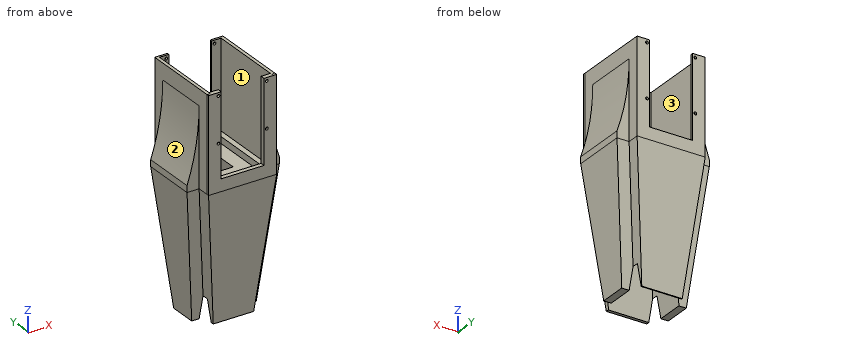
```python
from build123d import *
from build123d.topology import SkipClean

# Parameters (mm, degrees)
BOSS_EXTRUDE1_DEPTH      = 3
SKETCH2_W                = 25
SKETCH2_H                = 2
BOSS_EXTRUDE2_DEPTH      = 40
SKETCH3_R                = 0.625
CUT_EXTRUDE1_DEPTH       = 3
SKETCH4_R                = 0.625
CUT_EXTRUDE2_DEPTH       = 3
SKETCH7_W                = 19.5
SKETCH7_H                = 75
CUT_EXTRUDE5_DEPTH       = 40
SKETCH10_W               = 25
SKETCH10_H               = 3
BOSS_EXTRUDE4_DEPTH      = 10
SKETCH11_W               = 25
SKETCH11_H               = 3
BOSS_EXTRUDE5_DEPTH      = 10
SKETCH12_W               = 3
SKETCH12_H               = 25
BOSS_EXTRUDE6_DEPTH      = 10
SKETCH13_W               = 3
SKETCH13_H               = 25
BOSS_EXTRUDE7_DEPTH      = 10
SKETCH14_W               = 43
SKETCH14_H               = 35.95813892
BOSS_EXTRUDE11_DEPTH     = 3
SKETCH15_W               = 43
SKETCH15_H               = 35.95813892
BOSS_EXTRUDE12_DEPTH     = 3
SKETCH16_W               = 23
SKETCH16_H               = 28
CUT_EXTRUDE6_DEPTH       = 13
FILLET1_R                = 10
FILLET2_R                = 10
SKETCH19_W               = 28
SKETCH19_H               = 32
CUT_EXTRUDE9_DEPTH       = 40
CUT_EXTRUDE11_DEPTH      = 58.835974964
CUT_EXTRUDE11_DEPTH_BACK = 58.835974964
SKETCH20_W               = 25.25
SKETCH20_H               = 11.847644437
SKETCH20_W_2             = 25
SKETCH20_H_2             = 13.837487399
CUT_EXTRUDE13_DEPTH      = 56.982140009
CUT_EXTRUDE13_DEPTH_BACK = 56.982140009
SKETCH22_W               = 10
SKETCH22_H               = 25
FILLET3_R                = 100
FILLET4_R                = 100
SKETCH25_W               = 28
SKETCH25_H               = 2
CUT_EXTRUDE17_DEPTH      = 40
SKETCH27_R               = 0.625
BOSS_EXTRUDE14_DEPTH     = 1
SKETCH31_W               = 10
SKETCH31_H               = 10
BOSS_EXTRUDE16_DEPTH     = 60
BOSS_EXTRUDE16_TAPER     = 6


# Some blends are built 0.0001 mm under size
with BuildPart() as part:
    # Sketch1 → Boss-Extrude1 (new body)
    with BuildSketch(Plane.XY):
        Polygon((12.5, 12.5), (21, 12.5), (21, -12.5), (12.5, -12.5), (12.5, -18), (-12.5, -18), (-12.5, -12.5), (-21, -12.5), (-21, 12.5), (-12.5, 12.5), (-12.5, 18), (12.5, 18), align=None)
    extrude(amount=BOSS_EXTRUDE1_DEPTH)

    # Sketch2 → Boss-Extrude2 (add)
    with BuildSketch(Plane.XY.offset(3)):
        with Locations((0, 17)):
            Rectangle(SKETCH2_W, SKETCH2_H)
        with Locations((0, -17)):
            Rectangle(SKETCH2_W, SKETCH2_H)
    extrude(amount=BOSS_EXTRUDE2_DEPTH)

    # Sketch3 → Cut-Extrude1 (cut)
    with BuildSketch(Plane(origin=(0, 18, 0), x_dir=(1, 0, 0), z_dir=(0, 1, 0))):
        with Locations(Location((-11, -17.5, 0), (0, 0, 270))):
            Circle(SKETCH3_R)
        with Locations(Location((11, -17.5, 0), (0, 0, 270))):
            Circle(SKETCH3_R)
        with Locations(Location((-11, -41.5, 0), (0, 0, 270))):
            Circle(SKETCH3_R)
        with Locations(Location((11, -41.5, 0), (0, 0, 270))):
            Circle(SKETCH3_R)
    extrude(amount=-CUT_EXTRUDE1_DEPTH, mode=Mode.SUBTRACT)

    # Sketch4 → Cut-Extrude2 (cut)
    with BuildSketch(Plane(origin=(0, -16, 0), x_dir=(1, 0, 0), z_dir=(0, 1, 0))):
        with Locations(Location((-11, -41.5, 0), (0, 0, 270))):
            Circle(SKETCH4_R)
        with Locations(Location((11, -41.5, 0), (0, 0, 270))):
            Circle(SKETCH4_R)
        with Locations(Location((-11, -21, 0), (0, 0, 270))):
            Circle(SKETCH4_R)
        with Locations(Location((11, -21, 0), (0, 0, 270))):
            Circle(SKETCH4_R)
    extrude(amount=-CUT_EXTRUDE2_DEPTH, mode=Mode.SUBTRACT)

    # Sketch7 → Cut-Extrude5 (cut)
    with BuildSketch(Plane(origin=(0, 18, 0), x_dir=(1, 0, 0), z_dir=(0, 1, 0))):
        with Locations((0, -43)):
            Rectangle(SKETCH7_W, SKETCH7_H)
    extrude(amount=-CUT_EXTRUDE5_DEPTH, mode=Mode.SUBTRACT)

    # Sketch10 → Boss-Extrude4 (add)
    with BuildSketch(Plane(origin=(0, 18, 0), x_dir=(1, 0, 0), z_dir=(0, 1, 0))):
        with Locations((0, -1.5)):
            Rectangle(SKETCH10_W, SKETCH10_H)
    extrude(amount=BOSS_EXTRUDE4_DEPTH)

    # Sketch11 → Boss-Extrude5 (add)
    with BuildSketch(Plane.XZ.offset(18)):
        with Locations((0, 1.5)):
            Rectangle(SKETCH11_W, SKETCH11_H)
    extrude(amount=BOSS_EXTRUDE5_DEPTH)

    # Sketch12 → Boss-Extrude6 (add)
    with BuildSketch(Plane.ZY.offset(21)):
        with Locations((1.5, 0)):
            Rectangle(SKETCH12_W, SKETCH12_H)
    extrude(amount=BOSS_EXTRUDE6_DEPTH)

    # Sketch13 → Boss-Extrude7 (add)
    with BuildSketch(Plane(origin=(21, 0, 0), x_dir=(0, 0, -1), z_dir=(1, 0, 0))):
        with Locations((-1.5, 0)):
            Rectangle(SKETCH13_W, SKETCH13_H)
    extrude(amount=BOSS_EXTRUDE7_DEPTH)

    # Sketch14 → Boss-Extrude11 (add)
    with BuildSketch(Plane.ZY.offset(12.5)):
        with Locations((21.5, 0.02093054)):
            Rectangle(SKETCH14_W, SKETCH14_H)
    extrude(amount=BOSS_EXTRUDE11_DEPTH)

    # Sketch15 → Boss-Extrude12 (add)
    with BuildSketch(Plane(origin=(12.5, 0, 0), x_dir=(0, 0, -1), z_dir=(1, 0, 0))):
        with Locations((-21.5, 0.02093054)):
            Rectangle(SKETCH15_W, SKETCH15_H)
    extrude(amount=BOSS_EXTRUDE12_DEPTH)

    # Sketch16 → Cut-Extrude6 (cut)
    with BuildSketch(Plane(origin=(0, 0, 0), x_dir=(-1, 0, 0), z_dir=(0, 0, -1))):
        Rectangle(SKETCH16_W, SKETCH16_H)
    extrude(amount=-CUT_EXTRUDE6_DEPTH, mode=Mode.SUBTRACT)

    # Fillet1
    fillet1_edges = [part.edges().sort_by_distance(p)[0] for p in [
        (31, 12.5, 1.5),
    ]]
    fillet(fillet1_edges, radius=FILLET1_R)

    # Fillet2
    fillet2_edges = [part.edges().sort_by_distance(p)[0] for p in [
        (12.5, 28, 1.5),
        (-12.5, 28, 1.5),
        (-31, 12.5, 1.5),
        (12.5, -28, 1.5),
        (-31, -12.5, 1.5),
        (-12.5, -28, 1.5),
        (31, -12.5, 1.5),
    ]]
    fillet(fillet2_edges, radius=FILLET2_R - 0.0001)  # a hair under: the kernel refuses the full size

    # Sketch19 → Cut-Extrude9 (cut)
    with BuildSketch(Plane.XY.offset(43)):
        Rectangle(SKETCH19_W, SKETCH19_H)
    extrude(amount=-CUT_EXTRUDE9_DEPTH, mode=Mode.SUBTRACT)

    # Sketch20 → Cut-Extrude11 (cut, two sides: drawn at the far end of the back side and taken through both)
    with BuildSketch(Plane.XY.offset(3).offset(-CUT_EXTRUDE11_DEPTH_BACK)):
        with Locations((0, 23.923822218)):
            Rectangle(SKETCH20_W, SKETCH20_H)
        with Locations((0, -24.918743699)):
            Rectangle(SKETCH20_W_2, SKETCH20_H_2)
    extrude(amount=CUT_EXTRUDE11_DEPTH + CUT_EXTRUDE11_DEPTH_BACK, mode=Mode.SUBTRACT)

    # Sketch22 → Cut-Extrude13 (cut, two sides: drawn at the far end of the back side and taken through both)
    with BuildSketch(Plane(origin=(0, 0, 0), x_dir=(-1, 0, 0), z_dir=(0, 0, -1)).offset(-CUT_EXTRUDE13_DEPTH_BACK)):
        with Locations((26, 0)):
            Rectangle(SKETCH22_W, SKETCH22_H)
        with Locations((-26, 0)):
            Rectangle(SKETCH22_W, SKETCH22_H)
    extrude(amount=CUT_EXTRUDE13_DEPTH + CUT_EXTRUDE13_DEPTH_BACK, mode=Mode.SUBTRACT)

    # Fillet3
    # the kernel refuses this fillet: 100 mm, written as the material it adds along each edge
    with BuildSketch(Plane(origin=(-15.5, -12.5, 3), x_dir=(0, 0, 1), z_dir=(0, 1, 0))) as fillet3_piece_1:
        with BuildLine():
            CenterArc((32.707032883, -100), FILLET3_R, 90, 19.091052513)
            Line((0, -5.5), (0, 0))
            Line((0, 0), (32.707032883, 0))
        make_face()
    extrude(amount=25)

    # Fillet4
    # the kernel refuses this fillet: 100 mm, written as the material it adds along each edge
    with BuildSketch(Plane(origin=(15.5, -12.5, 3), x_dir=(1, 0, 0), z_dir=(0, 1, 0))) as fillet4_piece_1:
        with BuildLine():
            CenterArc((100, -32.707032883), FILLET4_R, 160.908947487, 19.091052513)
            Line((0, -32.707032883), (0, 0))
            Line((0, 0), (5.5, 0))
        make_face()
    extrude(amount=25)

    # Sketch25 → Cut-Extrude17 (cut)
    with BuildSketch(Plane.XY.offset(43)):
        with Locations((0, 16)):
            Rectangle(SKETCH25_W, SKETCH25_H)
        with Locations((0, -16)):
            Rectangle(SKETCH25_W, SKETCH25_H)
    extrude(amount=-CUT_EXTRUDE17_DEPTH, mode=Mode.SUBTRACT)

    # Sketch27 → Boss-Extrude14 (add)
    with SkipClean():  # the faces are left unmerged after this step: merging them gives an invalid solid
        with BuildSketch(Plane.XZ.offset(18)):
            Polygon((-15.5, 43), (-9.75, 43), (-9.75, 5.5), (9.75, 5.5), (9.75, 43), (15.5, 43), (15.5, 0), (-15.5, 0), align=None)
            with Locations(Location((-11, 41.5, 0), (0, 0, 90))):
                Circle(SKETCH27_R, mode=Mode.SUBTRACT)
            with Locations(Location((-11, 21, 0), (0, 0, 270))):
                Circle(SKETCH27_R, mode=Mode.SUBTRACT)
            with Locations(Location((11, 21, 0), (0, 0, 270))):
                Circle(SKETCH27_R, mode=Mode.SUBTRACT)
            with Locations(Location((11, 41.5, 0), (0, 0, 90))):
                Circle(SKETCH27_R, mode=Mode.SUBTRACT)
        extrude(amount=BOSS_EXTRUDE14_DEPTH)
    add(part.part.scale(1), mode=Mode.REPLACE)  # the faces are merged on a copy

    # Sketch31 → Boss-Extrude16 (add)
    with BuildSketch(Plane(origin=(0, 0, 0), x_dir=(-1, 0, 0), z_dir=(0, 0, -1))):
        Polygon((-15.5, 18), (-15.5, 12.5), (-21, 12.5), (-21, -12.5), (-15.5, -12.5), (-15.5, -19), (15.5, -19), (15.5, -12.5), (21, -12.5), (21, 12.5), (15.5, 12.5), (15.5, 18), align=None)
        Rectangle(SKETCH31_W, SKETCH31_H, mode=Mode.SUBTRACT)
    extrude(amount=BOSS_EXTRUDE16_DEPTH, taper=BOSS_EXTRUDE16_TAPER)


solid = part.part
```
Part model, mm, in its own coordinate system. Face numbers are marked on the shaded views. Coordinates: 2 decimals unless noted, no trailing zeros.
Item 1: Pin check, flat tips, straight feed: pin 1 (8 mm diameter, centred on x = -2, y = -14, fed in from -Z); pin 2 (0.8 mm diameter, centred on y = -18.5, z = 17, fed in from +X); pin 3 (1.7 mm diameter, centred on x = 17, z = 9.5, fed in from +Y); pin 4 (12 mm diameter, centred on y = 2, z = 31, fed in from -X). Stop position of each tip, or through.
Item 2: Probe line 1 (X direction, y = -18.25, z = 41.5) (3 decimals); line 2 (X direction, y = -16.5, z = 13.5); line 3 (X direction, y = -12, z = 1.5). List the from-to ranges inside material, lowest first.
Item 3: Mould opens along Y. For the marked faces 1, 2 and 3 say: released by +Y, released by -Y, zero draft, split by the parting line, or undercut.
Results found:
1. pin 1: stops at z = -60
1. pin 2: stops at x = 15.5
1. pin 3: stops at y = 12.5
1. pin 4: stops at x = -16.07
2. line 1: x = -15.5 to -11.625, -10.375 to -9.75, 9.75 to 10.375, 11.625 to 15.5
2. line 2: x = -15.5 to -14, 14 to 15.5
2. line 3: x = -21 to -11.5, 11.5 to 21
3. face 1: undercut
3. face 2: zero draft
3. face 3: undercut
